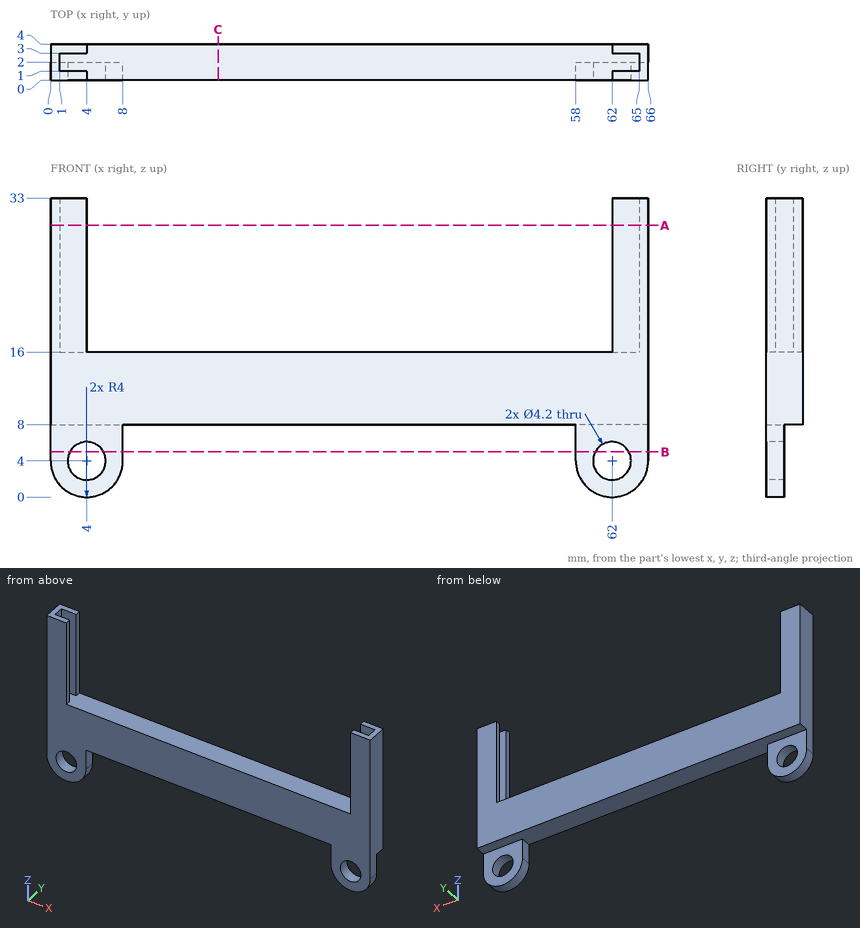
Print and shaded views of the part. All mm, measured from the part's lowest x, y and z. Coordinates: 2 decimals unless noted, no trailing zeros. Loops run counter-clockwise (first coordinate to the right, second up) from the corner with the lowest first, then second, coordinate; pieces in that order, holes last. Notation, with made-up numbers: (-16, 76.25) -> (41, 76.25) arc R22 ccw to (41, 110.25) -> close; hole circle Ø9 at (31, 56.5). An arc over 180 degrees is marked (long way). Use a Markdown table: item, result. Add a question column.
Item 1: Band-saw the part on C-C on x = 18.5. Write the cut outline in (y, z), plus the area to 3 significant figures.
Item 2: Band-saw the part on B-B on z = 5. Write the cut outline in (x, y).
Item 3: Flat gauge pins, fed straight in: P1, Ø1.5, axis at x = 17, y = 3.5, coming from the -Z side; P2, Ø1, axis at x = 36.5, y = 3, coming from the +Z side; P3, Ø2.5, axis at x = 2, z = 22.5, coming from the -Y side; P4, Ø4, axis at x = 61.5, z = 5.5, coming from the +Y side. Where does each tip first touch, or does it go through?
Item 4: Band-saw the part on A-A on z = 30. Write the cut outline in (x, y), plus the area to 3 significant figures.
Item 5: Probe probe 1 along Y at (x, z) = (3, 27); probe 2 along X at (y, z) = (0.4, 20.5); probe 3 along X at (y, z) = (1.9, 23). List the from-to ranges inside material, lowest first.
Geometry says:
| question | item | result |
|---|---|---|
| 1 | outline | (0, 8) -> (4, 8) -> (4, 16) -> (0, 16) -> close |
| 1 | area | 32.0 mm² |
| 2 | outline | (0, 0) -> (2.15, 0) -> (2.15, 2) -> (0, 2) -> close; (5.85, 0) -> (8, 0) -> (8, 2) -> (5.85, 2) -> close; (58, 0) -> (60.15, 0) -> (60.15, 2) -> (58, 2) -> close; (63.85, 0) -> (66, 0) -> (66, 2) -> (63.85, 2) -> close |
| 3 | P1 | z = 8 |
| 3 | P2 | z = 16 |
| 3 | P3 | y = 0 |
| 3 | P4 | y = 2 |
| 4 | outline | (0, 0) -> (4, 0) -> (4, 1) -> (1, 1) -> (1, 3) -> (4, 3) -> (4, 4) -> (0, 4) -> close; (62, 0) -> (66, 0) -> (66, 4) -> (62, 4) -> (62, 3) -> (65, 3) -> (65, 1) -> (62, 1) -> close |
| 4 | area | 20.0 mm² |
| 5 | probe 1 | 0 to 1, 3 to 4 |
| 5 | probe 2 | 0 to 4, 62 to 66 |
| 5 | probe 3 | 0 to 1, 65 to 66 |
